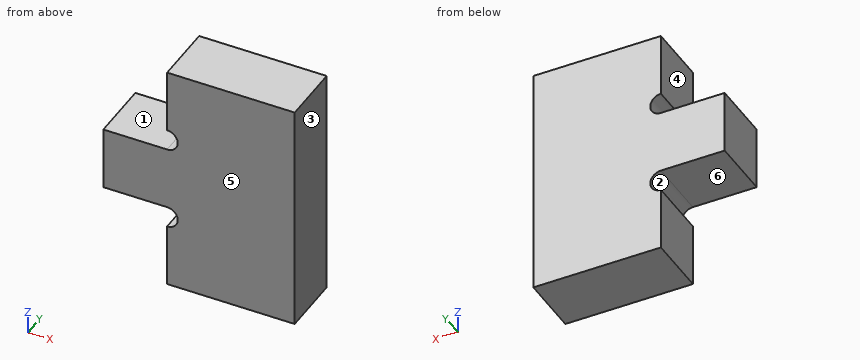
from build123d import *

# Parameters (mm, degrees)
BOSS_EXTRUDE1_DEPTH = 18.25625


with BuildPart() as part:
    # Sketch1 → Boss-Extrude1 (new body)
    with BuildSketch(Plane(origin=(0, 0, 0), x_dir=(1, 0, 0), z_dir=(0, 1, 0))):
        with BuildLine():
            Line((7.9375, 34.925), (7.9375, 15.875))
            ThreePointArc((7.9375, 15.875), (11.1125, 12.7), (7.9375, 9.525))
            Line((7.9375, 9.525), (-11.1125, 9.525))
            Line((-11.1125, 9.525), (-11.1125, -9.525))
            Line((-11.1125, -9.525), (7.9375, -9.525))
            ThreePointArc((7.9375, -9.525), (11.1125, -12.7), (7.9375, -15.875))
            Line((7.9375, -15.875), (7.9375, -34.925))
            Line((7.9375, -34.925), (46.0375, -34.925))
            Line((46.0375, -34.925), (46.0375, 34.925))
            Line((46.0375, 34.925), (7.9375, 34.925))
        make_face()
    extrude(amount=BOSS_EXTRUDE1_DEPTH)


solid = part.part
Work out the finished part from the listing and answer in its coordinate system (mm). Face numbers are marked on the shaded views. A direction names the side the tool comes from. Round coordinates to 2 decimals unless told otherwise and drop trailing zeros. Order: outer loops, then holes, each group sorted by start corner. A loop starts at its lowest first (then second) coordinate and runs counter-clockwise, first axis right, second up. Notation, with made-up numbers: M 46.25,26.5 L 93.25,26.5 A34 ccw 93.25,65.5 Z; hole C -22,-18.5 d11. An arc over 180 degrees is marked long. One line per item, written item: value.
Q1. Find section C-C on x = 0. Write down the section's boundary in (y, z) (3 decimals).
Derived:
outline: M 0,-9.525 L 18.256,-9.525 L 18.256,9.525 L 0,9.525 Z
Q2. Flat-ended cylindrical pins translate along their axes: pin 1 (4 mm diameter, centred on x = 39, z = 23, fed in from -Y); pin 2 (3 mm diameter, centred on y = 14, z = -20.5, fed in from -X); pin 3 (10 mm diameter, centred on x = -0.5, y = 16, fed in from -Z) (3 decimals). Find the tip coordinate at first contact, or state that the pin passes through.
Derived:
pin 1: y = 0
pin 2: x = 7.94
pin 3: z = -9.525
Q3. For the marked faces 4, 5 and 6, determine the directions among +Z, -Z, +X, -X, +Y, -Y from which every point of the face is accessible in a straight line to the end or side of a thin tool.
Derived:
face 4: +Z, -X, +Y, -Y
face 5: +Z, -Z, +X, -X, -Y
face 6: -Z, -X, +Y, -Y
Q4. Determine the mould class of the marked faces 1, 2 and 3 for opening direction Z: released by +Z, released by -Z, zero draft, split by the parting line, or undercut.
Derived:
face 1: released by +Z
face 2: undercut
face 3: zero draft
Q5. Straight lines are drawn through the part: line 1 (X direction, y = 9.25, z = -26); line 2 (X direction, y = 3.5, z = -12.5); line 3 (Z direction, x = 6, y = 6.75) (3 decimals). For each, find the intervals that lie inside material, in ascending order.
Derived:
line 1: 7.94 to 46.04
line 2: 11.11 to 46.04
line 3: -9.525 to 9.525
Q6. Find section B-B on z = -12.7. Write down the section's boundary in (x, y).
Derived:
outline: M 11.11,0 L 46.04,0 L 46.04,18.26 L 11.11,18.26 Z
